```python
from build123d import *

# Parameters (mm, degrees)
SKETCH1_R           = 6.5
BOSS_EXTRUDE1_DEPTH = 6
SKETCH3_R           = 6.5
SKETCH3_R_2         = 1
BOSS_EXTRUDE2_DEPTH = 4
SKETCH4_R           = 2.5
CUT_EXTRUDE1_DEPTH  = 2
FILLET1_R           = 0.4


with BuildPart() as part:
    # Sketch1 → Boss-Extrude1 (new body)
    with BuildSketch(Plane(origin=(0, 0, 0), x_dir=(1, 0, 0), z_dir=(0, 1, 0))):
        with Locations(Location((0, 0, 0), (0, 0, 270))):
            Circle(SKETCH1_R)
        Polygon((5.05, -2.915618859), (5.05, 2.915618859), (0, 5.831237719), (-5.05, 2.915618859), (-5.05, -2.915618859), (0, -5.831237719), align=None, mode=Mode.SUBTRACT)
    extrude(amount=BOSS_EXTRUDE1_DEPTH)

    # Sketch3 → Boss-Extrude2 (add)
    with BuildSketch(Plane(origin=(0, 6, 0), x_dir=(1, 0, 0), z_dir=(0, 1, 0))):
        with Locations(Location((0, 0, 0), (0, 0, 270))):
            Circle(SKETCH3_R)
        with Locations(Location((0, 0, 0), (0, 0, 270))):
            Circle(SKETCH3_R_2, mode=Mode.SUBTRACT)
    extrude(amount=BOSS_EXTRUDE2_DEPTH)

    # Sketch4 → Cut-Extrude1 (cut)
    with BuildSketch(Plane(origin=(0, 10, 0), x_dir=(1, 0, 0), z_dir=(0, 1, 0))):
        with Locations(Location((0, 0, 0), (0, 0, 270))):
            Circle(SKETCH4_R)
    extrude(amount=-CUT_EXTRUDE1_DEPTH, mode=Mode.SUBTRACT)

    # Fillet1
    fillet1_edges = [part.edges().sort_by_distance(p)[0] for p in [
        (0, 10, -2.5),
    ]]
    fillet(fillet1_edges, radius=FILLET1_R)


solid = part.part
```
Geometry: final body of the model. Coordinates: model frame, mm. A direction names the side the tool comes from. Round coordinates to 2 decimals unless told otherwise and drop trailing zeros. Order: outer loops, then holes, each group sorted by start corner. A loop starts at its lowest first (then second) coordinate and runs counter-clockwise, first axis right, second up. Notation, with made-up numbers: (84, 33.25) -> (107, 33.25) arc R30 cw to (107, 67.25) -> close; hole circle Ø2 at (67.5, 64). An arc over 180 degrees is marked (long way). Use CSV: the item, a comma, the result in double quotes. Start each with the question number.
1) Section D-D (x = -4). Return the cut outline in (y, z).
2) Section C-C (z = -3.25). Return the cut outline in (x, y).
3) Draft query along Z for faces 1 (the face through (-1, 10, 3)), 2 (the face through (-3.955, 4.93, -5.158)), 3 (the face through (-1, 7, 0)). Return one class per face: +Z half, -Z half, draft (parallel to the pull), parting line (faces both ways), or undercut.
4) Set-up query: faces 4 (the face through (2.56, 2.958, -4.353)), 5 (the face through (2, 0, -5)), 6 (the face through (-1, 8, 1)). Return all of +Z, -Z, +X, -X, +Y, -Y with unobstructed straight access to the full face (end or side cutting, diameter ignored); none if empty.
5) Section A-A (z = 0). Return the cut outline in (x, y).
6) Material intervals for line 1 along X through (y, z) = (7.5, 0); line 2 along Y through (x, z) = (5, -1.5); line 3 along X through (y, z) = (8.65, 0), sorted ascending. Write a range as from..to.
7) First-contact query: pin 1 Ø2.5 at (x, z) = (0, 0) entering from +Y; pin 2 Ø1 at (y, z) = (7, 1) entering from +X; pin 3 Ø4.5 at (y, z) = (3, -0.5) entering from -X; pin 4 Ø5 at (y, z) = (1.5, 4) entering from -X. Flat tips, straight axial feed; report the tip coordinate or a pass-through.
8) Section B-B (y = 1.75). Return the cut outline in (x, z), and give its area (3 significant figures).
Returned:
1,outline,"(0, -5.12) -> (10, -5.12) -> (10, 5.12) -> (0, 5.12) -> (0, 3.52) -> (6, 3.52) -> (6, -3.52) -> (0, -3.52) -> close"
2,outline,"(-5.63, 0) -> (-4.47, 0) -> (-4.47, 6) -> (4.47, 6) -> (4.47, 0) -> (5.63, 0) -> (5.63, 10) -> (-5.63, 10) -> close"
3,face 1,"draft"
3,face 2,"parting line"
3,face 3,"undercut"
4,face 4,"-Y"
4,face 5,"+Z, -Z, +X, -X, -Y"
4,face 6,"+Y"
5,outline,"(-6.5, 0) -> (-5.05, 0) -> (-5.05, 6) -> (-1, 6) -> (-1, 8) -> (-2.5, 8) -> (-2.5, 9.6) arc R0.4 ccw to (-2.9, 10) -> (-6.5, 10) -> close; (1, 6) -> (5.05, 6) -> (5.05, 0) -> (6.5, 0) -> (6.5, 10) -> (2.9, 10) arc R0.4 ccw to (2.5, 9.6) -> (2.5, 8) -> (1, 8) -> close"
6,line 1,"x = -6.5..-1, 1..6.5"
6,line 2,"y = 6..10"
6,line 3,"x = -6.5..-2.5, 2.5..6.5"
7,pin 1,"stops at y = 8"
7,pin 2,"stops at x = 6.48"
7,pin 3,"stops at x = -6.5"
7,pin 4,"stops at x = -6.32"
8,outline,"circle Ø13 at (0, 0); hole (-5.05, -2.92) -> (0, -5.83) -> (5.05, -2.92) -> (5.05, 2.92) -> (0, 5.83) -> (-5.05, 2.92) -> close"
8,area,"44.4 mm²"
